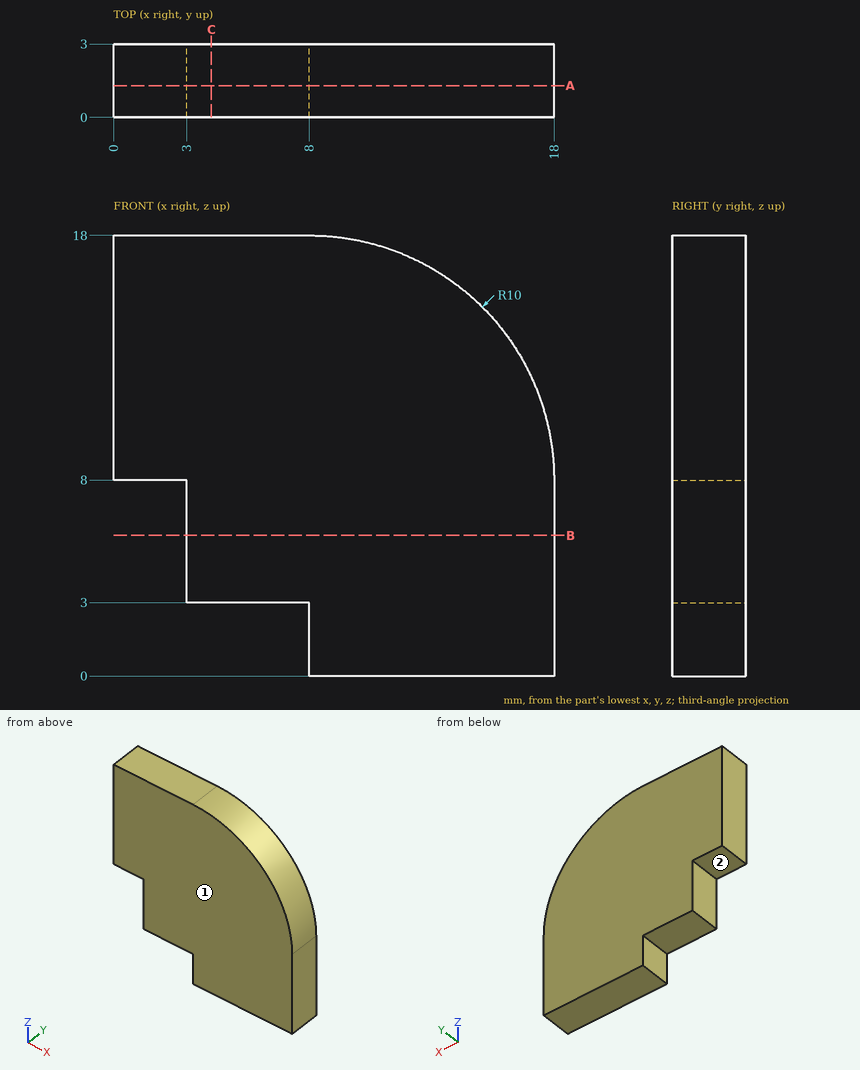
Study the drawing (mm; zero at the part's minimum x, y, z) and answer. A direction names the side the tool comes from. Give positions to 0.01 mm unless a question says otherwise; leave off trailing zeros. Write each loop counter-clockwise with the first axis right and the second up, starting at its lowest first coordinate (ties: lowest second). Pieces come first, ordered by that corner, then holes. Notation, with made-up numbers: (-35, -25.75) -> (-14, -25.75) arc R26 cw to (-14, 5.25) -> close; hole circle Ø1 at (-21, 53). An arc over 180 degrees is marked (long way). Answer in a Markdown table with one row per item.
1) Each of these flat-tipped pins is pushed along its axis until it touches: pin 1 Ø0.9 at (y, z) = (1, 4.5) entering from -X; pin 2 Ø10 at (x, z) = (2.5, 13) entering from -Y; pin 3 Ø0.9 at (y, z) = (1.5, 1) entering from -X; pin 4 Ø0.9 at (x, y) = (5, 1) entering from -Z. Where does it stop, or does it pass through?
Results list:
| item | result |
|---|---|
| pin 1 | x = 3 |
| pin 2 | y = 0 |
| pin 3 | x = 8 |
| pin 4 | z = 3 |
2) Section C-C on x = 4 is taken. Give the vertices of the cut face in (y, z), plus the area to 3 significant figures.
Results list:
| item | result |
|---|---|
| outline | (0, 3) -> (3, 3) -> (3, 18) -> (0, 18) -> close |
| area | 45.0 mm^2 |
3) Section B-B on z = 5.75 is taken. Give the vertices of the cut face in (x, y), plus the area to 3 significant figures.
Results list:
| item | result |
|---|---|
| outline | (3, 0) -> (18, 0) -> (18, 3) -> (3, 3) -> close |
| area | 45.0 mm^2 |
4) A tool of negligible diameter and unlimited length cuts with its end or side. For the marked faces 1 and 2, from which of +Z, -Z, +X, -X, +Y, -Y can it reach the whole face along a straight path? Write none if from no direction.
Results list:
| item | result |
|---|---|
| face 1 | +Z, -Z, +X, -X, -Y |
| face 2 | -Z, -X, +Y, -Y |
5) Straight lines are drawn through the part: line 1 (Z direction, x = 1.5, y = 0.8); line 2 (X direction, y = 2.5, z = 4.5); line 3 (X direction, y = 1.6, z = 11.5). For each, find the intervals that lie inside material, in ascending order. Write a range as [from, to].
Results list:
| item | result |
|---|---|
| line 1 | [8, 18] |
| line 2 | [3, 18] |
| line 3 | [0, 17.37] |
6) Section A-A on y = 1.3 is taken. Give the vertices of the cut face in (x, z).
Results list:
| item | result |
|---|---|
| outline | (0, 8) -> (3, 8) -> (3, 3) -> (8, 3) -> (8, 0) -> (18, 0) -> (18, 8) arc R10 ccw to (8, 18) -> (0, 18) -> close |
